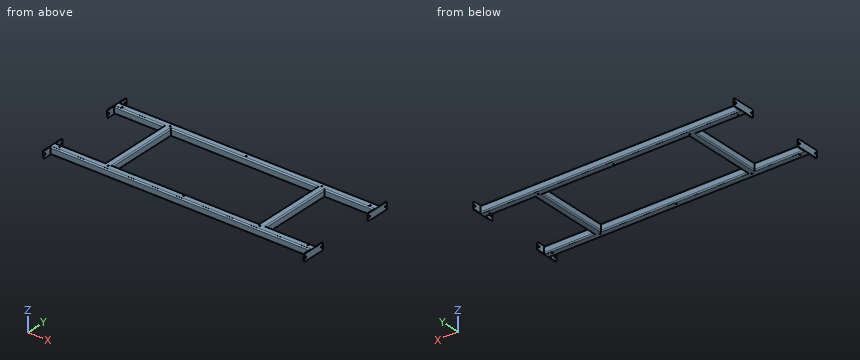
```python
from build123d import *

# Parameters (mm, degrees)
F0_W      = 614
F0_H      = 309
F1_DEPTH  = 30
F2_T      = -3
F3_W      = 35
F3_H      = 30
F3_W_2    = 30
F3_W_3    = 24
F3_H_2    = 24
F4_DEPTH  = 3
F6_SIZE   = 2
F7_R      = 5
F8_R      = 3
F10_D     = 6.4
F10_DEPTH = 3
F10_TIP   = 1.9227539809
F13_D     = 5


with BuildPart() as f1:
    # F0 (on Top) → F1 (new body)
    with BuildSketch(Plane.XY):
        Polygon((-337, -154.5), (-544.5, -154.5), (-544.5, -184.5), (544.5, -184.5), (544.5, -154.5), (337, -154.5), (337, 154.5), (544.5, 154.5), (544.5, 184.5), (-544.5, 184.5), (-544.5, 154.5), (-337, 154.5), align=None)
        Rectangle(F0_W, F0_H, mode=Mode.SUBTRACT)
    extrude(amount=-F1_DEPTH)

    # F2
    f2_openings = [f1.faces().sort_by_distance(p)[0] for p in [
        (-544.5, -169.5, -15),
        (-544.5, 169.5, -15),
        (544.5, 169.5, -15),
        (544.5, -169.5, -15),
    ]]
    offset(amount=F2_T, openings=f2_openings, kind=Kind.INTERSECTION)

    # F7
    f7_edges = [f1.edges().sort_by_distance(p)[0] for p in [
        (0, -184.5, -30),
        (-440.75, -154.5, -30),
        (-337, 0, -30),
        (-307, 0, -30),
        (0, -154.5, -30),
        (-440.75, 154.5, -30),
        (0, 184.5, -30),
        (307, 0, -30),
        (337, 0, -30),
        (0, 154.5, -30),
        (440.75, 154.5, -30),
        (0, 184.5, 0),
        (-440.75, 154.5, 0),
        (0, 154.5, 0),
        (-337, 0, 0),
        (-307, 0, 0),
        (-440.75, -154.5, 0),
        (0, -154.5, 0),
        (307, 0, 0),
        (337, 0, 0),
        (440.75, -154.5, 0),
        (440.75, 154.5, 0),
        (440.75, -154.5, -30),
        (0, -184.5, 0),
    ]]
    fillet(f7_edges, radius=F7_R)

    # F8
    f8_edges = [f1.edges().sort_by_distance(p)[0] for p in [
        (-439.25, 157.5, -3),
        (-439.25, 157.5, -27),
        (0, 181.5, -27),
        (0, 181.5, -3),
        (0, -181.5, -3),
        (439.25, -157.5, -3),
        (439.25, -157.5, -27),
        (0, -181.5, -27),
    ]]
    fillet(f8_edges, radius=F8_R)



with BuildPart() as f4:
    # F3 (on face) → F4 (new body)
    with BuildSketch(Plane(origin=(-544.5, 0, 0), x_dir=(0, -1, 0), z_dir=(-1, 0, 0))):
        with Locations((202, -15)):
            Rectangle(F3_W, F3_H)
        with Locations((137, -15)):
            Rectangle(F3_W, F3_H)
        with Locations((169.5, -15)):
            Rectangle(F3_W_2, F3_H)
        with Locations((169.5, -15)):
            Rectangle(F3_W_3, F3_H_2, mode=Mode.SUBTRACT)
        with Locations((169.5, -15)):
            Rectangle(F3_W_3, F3_H_2)
    extrude(amount=F4_DEPTH)

    # F6
    f6_edges = [f4.edges().sort_by_distance(p)[0] for p in [
        (-546, -219.5, -30),
        (-546, -219.5, 0),
        (-546, -119.5, -30),
        (-546, -119.5, 0),
    ]]
    chamfer(f6_edges, length=F6_SIZE)

    # F10
    with Locations(Plane(origin=(-547.5, 0, 0), x_dir=(0, -1, 0), z_dir=(-1, 0, 0))):
        with Locations((127, -15), (212, -15)):
            Hole(F10_D / 2, depth=F10_DEPTH)
            with Locations((0, 0, -(F10_DEPTH + F10_TIP / 2))):  # 118° drill point
                Cone(0, F10_D / 2, F10_TIP, mode=Mode.SUBTRACT)


with BuildPart() as f11_1:
    # F11: instance of F4
    add(f4.part.mirror(Plane.YZ))


with BuildPart() as f1_1:
    add(f1.part)

    add(f4.part)  # F12 merges F4

    add(f11_1.part)  # F12 merges F11_1
    # F12: F4, F11_1 across plane
    add(f4.part.mirror(Plane.XZ))
    add(f11_1.part.mirror(Plane.XZ))

    # F13 (through all)
    with Locations(Plane.XY):
        with Locations((-520, 165), (-317.5, 165), (0, 165), (317.5, 165), (520, 165), (520, -165), (317.5, -165), (0, -165), (-317.5, -165), (-520, -165)):
            Hole(F13_D / 2)


solid = f1_1.part
```
Input: part model. Units: mm. Frame: model coordinates. Give positions to 0.01 mm unless a question says otherwise; leave off trailing zeros. Order: outer loops, then holes, each group sorted by start corner. A loop starts at its lowest first (then second) coordinate and runs counter-clockwise, first axis right, second up. Notation, with made-up numbers: (-3.75, 11.25) -> (36.25, 11.25) arc R8 ccw to (36.25, 26.25) -> close; hole circle Ø1 at (7.5, -24). An arc over 180 degrees is marked (long way). Write each question's results on one line, items separated by ' | '. Start each with the question number.
Item 1: Cut plane B-B on y = -15.5. Return the cut outline in (x, z), then the cut area to 3 significant figures.
Item 2: Line query: line 1 (Y direction, x = 545, z = -15); line 2 (X direction, y = -165, z = -2.4); line 3 (X direction, y = 156.5, z = -12). Output: solid intervals per line, ascending.
Item 3: Cut plane A-A on x = -169.5. Return the cut outline in (y, z), then the cut area to 3 significant figures.
Item 4: Contact query for flat-ended pins moving along their axis: P1, Ø1.5, axis at x = -181, z = -4, coming from the +Y side; P2, Ø3, axis at y = 93, z = -5.5, coming from the +X side; P3, Ø16, axis at x = 449.5, z = -14, coming from the -Y side; P4, Ø8.5, axis at y = -212, z = -15, coming from the +X side. Output: stop coordinate, or through.
Item 5: Cut plane C-C on x = 436. Give the number of separate pieces and of enclosed holes in the cut face, then the cut area to 3 significant figures.
Established:
1) outline: (-337, -25) arc R5 ccw to (-332, -30) -> (-312, -30) arc R5 ccw to (-307, -25) -> (-307, -5) arc R5 ccw to (-312, 0) -> (-332, 0) arc R5 ccw to (-337, -5) -> close; (307, -25) arc R5 ccw to (312, -30) -> (332, -30) arc R5 ccw to (337, -25) -> (337, -5) arc R5 ccw to (332, 0) -> (312, 0) arc R5 ccw to (307, -5) -> close; hole (-334, -27) -> (-310, -27) -> (-310, -3) -> (-334, -3) -> close; hole (310, -27) -> (334, -27) -> (334, -3) -> (310, -3) -> close | area: 605 mm^2
2) line 1: -219.5 to -215.2, -208.8 to -130.2, -123.8 to -119.5, 119.5 to 123.8, 130.2 to 208.8, 215.2 to 219.5 | line 2: -547.5 to -522.5, -517.5 to -320, -315 to -2.5, 2.5 to 315, 320 to 517.5, 522.5 to 547.5 | line 3: -547.5 to -334, -310 to 310, 334 to 547.5
3) outline: (-184.5, -25) arc R5 ccw to (-179.5, -30) -> (-159.5, -30) arc R5 ccw to (-154.5, -25) -> (-154.5, -5) arc R5 ccw to (-159.5, 0) -> (-179.5, 0) arc R5 ccw to (-184.5, -5) -> close; (154.5, -25) arc R5 ccw to (159.5, -30) -> (179.5, -30) arc R5 ccw to (184.5, -25) -> (184.5, -5) arc R5 ccw to (179.5, 0) -> (159.5, 0) arc R5 ccw to (154.5, -5) -> close; hole (-181.5, -24) arc R3 ccw to (-178.5, -27) -> (-157.5, -27) -> (-157.5, -3) -> (-178.5, -3) arc R3 ccw to (-181.5, -6) -> close; hole (157.5, -27) -> (178.5, -27) arc R3 ccw to (181.5, -24) -> (181.5, -6) arc R3 ccw to (178.5, -3) -> (157.5, -3) -> close | area: 613 mm^2
4) P1: y = 184.49 | P2: x = 337 | P3: y = -184.5 | P4: x = 547.5
5) separate pieces: 2 | enclosed holes: 2 | area: 617 mm^2
